Geometry: final body of the model. Coordinates: model frame, mm. A direction names the side the tool comes from. Round coordinates to 2 decimals unless told otherwise and drop trailing zeros. Write each loop counter-clockwise with the first axis right and the second up, starting at its lowest first coordinate (ties: lowest second). Pieces come first, ordered by that corner, then holes. Notation, with made-up numbers: M -28,14 L 11,14 A19 ccw 11,21 Z; hole C -27,-35 d11. An arc over 180 degrees is marked long. Use one line per item in the form item = value. Start each with the question number.
from build123d import *

# Parameters (mm, degrees)
SKETCH_R        = 5.5
SKETCH_R_2      = 10
SKETCH_R_3      = 2
SKETCH_W        = 50
SKETCH_H        = 21
SKETCH_W_2      = 23
SKETCH_H_2      = 38.5
PAD_DEPTH       = 3
FILLET_R        = 5
FILLET001_R     = 15
SKETCH001_R     = 1.25
SKETCH001_R_2   = 2.5
POCKET_DEPTH    = 3.001
FILLET002_R     = 2
FILLET003_R     = 2
SKETCH002_W     = 4
SKETCH002_H     = 21
POCKET001_DEPTH = 3.001


with BuildPart() as part:
    # Sketch → Pad (new body)
    with BuildSketch(Plane.XY):
        with BuildLine():
            Line((0, 15), (0, 25))
            ThreePointArc((15, 40), (4.393398, 35.606602), (0, 25))
            Line((15, 40), (42, 40))
            ThreePointArc((42, 40), (52.606602, 44.393398), (57, 55))
            Line((57, 55), (57, 120))
            ThreePointArc((57, 120), (52.606602, 130.606602), (42, 135))
            Line((42, 135), (-4, 135))
            ThreePointArc((-4, 135), (-14.606602, 130.606602), (-19, 120))
            Line((-19, 120), (-19, 83))
            ThreePointArc((-48.374211, 78.71257), (-31.833571, 68.157272), (-19, 83))
            ThreePointArc((-48.374211, 78.71257), (-56.140556, 83.224713), (-63.9069, 78.71257))
            ThreePointArc((-130, 65), (-93.858369, 56.938332), (-63.9069, 78.71257))
            ThreePointArc((-130, 65), (-134.416408, 59.708204), (-136, 53))
            Line((-136, 53), (-136, 15))
            ThreePointArc((-136, 15), (-131.606602, 4.393398), (-121, 0))
            Line((-121, 0), (-15, 0))
            ThreePointArc((-15, 0), (-4.393398, 4.393398), (0, 15))
        make_face()
        with Locations((-118, 18)):
            Circle(SKETCH_R, mode=Mode.SUBTRACT)
        with Locations((-18, 18)):
            Circle(SKETCH_R, mode=Mode.SUBTRACT)
        with Locations((38, 119.5)):
            Circle(SKETCH_R_2, mode=Mode.SUBTRACT)
        with Locations((38, 90.5)):
            Circle(SKETCH_R_2, mode=Mode.SUBTRACT)
        with Locations((-86.944694, 45.077738)):
            Circle(SKETCH_R_3, mode=Mode.SUBTRACT)
        with Locations((-57.480095, 69.07435)):
            Circle(SKETCH_R_3, mode=Mode.SUBTRACT)
        with Locations((-38.535401, 45.812824)):
            Circle(SKETCH_R_3, mode=Mode.SUBTRACT)
        with Locations((-68, 21.816212)):
            Circle(SKETCH_R_3, mode=Mode.SUBTRACT)
        with Locations((-68, 47.675445)):
            Circle(SKETCH_R_3, mode=Mode.SUBTRACT)
        with Locations((-20, 54)):
            Circle(SKETCH_R_3, mode=Mode.SUBTRACT)
        with Locations((19, 64.5)):
            Rectangle(SKETCH_W, SKETCH_H, mode=Mode.SUBTRACT)
        with Locations((0, 102.75)):
            Rectangle(SKETCH_W_2, SKETCH_H_2, mode=Mode.SUBTRACT)
    extrude(amount=PAD_DEPTH)

    # Fillet
    fillet_edges = [part.edges().sort_by_distance(p)[0] for p in [
        (-48.374211, 78.71257, 1.5),
    ]]
    fillet(fillet_edges, radius=FILLET_R)

    # Fillet001
    fillet001_edges = [part.edges().sort_by_distance(p)[0] for p in [
        (-130, 65, 1.5),
    ]]
    fillet(fillet001_edges, radius=FILLET001_R)

    # Sketch001 (on Face38 of Fillet001) → Pocket (cut, through all)
    with BuildSketch(Plane.XY.offset(3)):
        with Locations((48, 119.5)):
            Circle(SKETCH001_R)
        with Locations((48, 90.5)):
            Circle(SKETCH001_R)
        with Locations((-7, 56)):
            Circle(SKETCH001_R_2)
        with Locations((45, 56)):
            Circle(SKETCH001_R_2)
    extrude(amount=-POCKET_DEPTH, mode=Mode.SUBTRACT)

    # Fillet002
    fillet002_edges = [part.edges().sort_by_distance(p)[0] for p in [
        (44, 58.291288, 1.5),
        (-6, 58.291288, 1.5),
    ]]
    fillet(fillet002_edges, radius=FILLET002_R)

    # Fillet003
    fillet003_edges = [part.edges().sort_by_distance(p)[0] for p in [
        (-5.5, 54, 1.5),
        (43.5, 54, 1.5),
    ]]
    fillet(fillet003_edges, radius=FILLET003_R)

    # Sketch002 (on Face46 of Fillet003) → Pocket001 (cut, through all)
    with BuildSketch(Plane.XY.offset(3)):
        with Locations((38, 119.5)):
            Rectangle(SKETCH002_W, SKETCH002_H)
        with Locations((38, 90.5)):
            Rectangle(SKETCH002_W, SKETCH002_H)
    extrude(amount=-POCKET001_DEPTH, mode=Mode.SUBTRACT)


solid = part.part
1. Contact query for flat-ended pins moving along their axis: pin 1 (1 mm diameter, centred on x = 20, z = 2.5, fed in from -Y); pin 2 (1.5 mm diameter, centred on y = 67, z = 1.5, fed in from -X); pin 3 (3.5 mm diameter, centred on x = -38.54, y = 45.81, fed in from +Z); pin 4 (0.8 mm diameter, centred on y = 129.5, z = 2, fed in from +X). Output: stop coordinate, or through.
2. Section query C-C (y = 9). Return loops of the section in (x, z).
3. Ray query, probe 1 along Y at (x, z) = (9.5, 1.9); probe 2 along X at (y, z) = (104.5, 2.7); probe 3 along Y at (x, z) = (42, 0.65). Return the intervals inside material, ascending.
4. Section query A-A (x = -87). Return loops of the section in (y, z), then the cut area to 3 significant figures.
5. Section query B-B (z = 2.1). Give the number of separate pieces and of enclosed holes in the cut face, then the cut area to 3 significant figures.
6. Pull-direction query (Y, two-part tool) for faces 1 (the face through (47.33, 55.09, 1.52)), 2 (the face through (-41, 53, 0)), 3 (the face through (-14.49, 130.72, 1.48)); classes: released by +Y, released by -Y, zero draft, split by the parting line, or undercut.
7. Set-up query: faces 4 (the face through (28, 119.7, 1.5)), 5 (the face through (-31.856, 68.154, 1.479)). Return all of +Z, -Z, +X, -X, +Y, -Y with unobstructed straight access to the full face (end or side cutting, diameter ignored); none if empty.
Checks:
q1.pin_1 = 40
q1.pin_2 = -74.41
q1.pin_3 = through
q1.pin_4 = 53.92
q2.outline = M -134.75,0 L -1.25,0 L -1.25,3 L -134.75,3 Z
q3.probe_1 = 38.96 to 54, 75 to 83.5, 122 to 135
q3.probe_2 = -19 to -11.5, 11.5 to 57
q3.probe_3 = 40 to 54, 75 to 81.33, 99.67 to 110.33, 128.67 to 135
q4.outline = M 0,0 L 43.08,0 L 43.08,3 L 0,3 Z; M 47.08,0 L 58.94,0 L 58.94,3 L 47.08,3 Z
q4.area = 165 mm^2
q5.separate_pieces = 1
q5.enclosed_holes = 12
q5.area = 12,600 mm^2
q6.face_1 = undercut
q6.face_2 = zero draft
q6.face_3 = released by +Y
q7.face_4 = +Z, -Z
q7.face_5 = +Z, -Z, +Y
